Part model, mm, in its own coordinate system. A direction names the side the tool comes from. Coordinates: 2 decimals unless noted, no trailing zeros. Write each loop counter-clockwise with the first axis right and the second up, starting at its lowest first coordinate (ties: lowest second). Pieces come first, ordered by that corner, then holes. Notation, with made-up numbers: (25.25, 53.5) - (40.25, 53.5) arc R34 ccw to (40.25, 91.5) - close; hole circle Ø3 at (2, 16.5). An arc over 180 degrees is marked (long way). Write each question's results on one line, items separated by ' | '.
from build123d import *

# Parameters (mm, degrees)
F0_W      = 23
F0_H      = 18
F1_DEPTH  = 10
F2_W      = 6
F2_H      = 6
F2_H_2    = 5
F3_DEPTH  = 2.5
F4_R      = 1.19
F5_DEPTH  = 5
F6_W      = 14
F6_H      = 14
F7_DEPTH  = 5
F8_R      = 1.15
F8_R_2    = 1
F9_DEPTH  = 5
F10_W     = 23
F10_H     = 2.5
F11_DEPTH = 2


with BuildPart() as f1:
    # F0 (on Top) → F1 (new body)
    with BuildSketch(Plane.XY):
        Rectangle(F0_W, F0_H)
    extrude(amount=F1_DEPTH)

    # F2 (on face) → F3 (join)
    with BuildSketch(Plane(origin=(0, 0, 0), x_dir=(1, 0, 0), z_dir=(0, 0, -1))):
        with Locations((-8.5, 6)):
            Rectangle(F2_W, F2_H)
        with Locations((8.5, 6.5)):
            Rectangle(F2_W, F2_H_2)
    extrude(amount=F3_DEPTH)

    # F4 (on face) → F5 (join)
    with BuildSketch(Plane(origin=(0, 0, -2.5), x_dir=(1, 0, 0), z_dir=(0, 0, -1))):
        with Locations((-8.5, 6)):
            Circle(F4_R)
    extrude(amount=F5_DEPTH)

    # F6 (on face) → F7 (cut)
    with BuildSketch(Plane.XY.offset(10)):
        with Locations((0, -2)):
            Rectangle(F6_W, F6_H)
    extrude(amount=-F7_DEPTH, mode=Mode.SUBTRACT)

    # F8 (on face) → F9 (join)
    with BuildSketch(Plane.XY.offset(10)):
        with Locations((-8.9, -6.5)):
            Circle(F8_R)
        with Locations((8.9, -6.5)):
            Circle(F8_R_2)
    extrude(amount=F9_DEPTH)

    # F10 (on face) → F11 (cut)
    with BuildSketch(Plane.XY.offset(10)):
        with Locations((0, 7.75)):
            Rectangle(F10_W, F10_H)
    extrude(amount=-F11_DEPTH, mode=Mode.SUBTRACT)


solid = f1.part
(1) 3-axis set-ups, long thin cutter, end or side, ignore diameter. For faces 1 (the cylindrical face through (7.9, -6.5, 12.5)), 2 (the flat face through (0, 6.5, 9)), 3 (the flat face through (5.5, -6, -1)), 4 (the flat face through (-7, -6, -2.5)), 5 (the flat face through (0, 5, 8)): which of +Z, -Z, +X, -X, +Y, -Y reach the whole face in a straight line?
Return value:
face 1: +Z | face 2: +Z, +X, -X, +Y | face 3: -Z, +Y, -Y | face 4: -Z | face 5: +Z, -Y
(2) Saw through at B-B on x = -1. Write the cut outline in (y, z), then the cut area to 3 significant figures.
Return value:
outline: (-9, 0) - (9, 0) - (9, 8) - (6.5, 8) - (6.5, 10) - (5, 10) - (5, 5) - (-9, 5) - close | area: 105 mm^2
(3) Saw through at D-D on x = -6. Write the cut outline in (y, z).
Return value:
outline: (-9, -2.5) - (-3, -2.5) - (-3, 0) - (9, 0) - (9, 8) - (6.5, 8) - (6.5, 10) - (5, 10) - (5, 5) - (-9, 5) - close
(4) Flat gauge pins, fed straight in: P1, Ø6, axis at x = -3, y = -5.5, coming from the -Z side; P2, Ø8, axis at x = 2.5, y = 0.5, coming from the +Z side; P3, Ø8, axis at x = 5, y = -3.5, coming from the +Z side; P4, Ø0.8, axis at x = 7, z = -1, coming from the +Y side. Where does each tip first touch, or does it go through?
Return value:
P1: stops at z = -2.5 | P2: stops at z = 5 | P3: stops at z = 15 | P4: stops at y = -4
(5) Two-plate mould, pull along Y, no slides. Class faces 6 (the cylindrical face through (-9.748, -5.723, 12.465)), 7 (the flat face through (-5.5, -6, -1)), 8 (the flat face through (8, -4, -1)): released by +Y, released by -Y, zero draft, split by the parting line, or undercut.
Return value:
face 6: split by the parting line | face 7: zero draft | face 8: released by +Y
(6) Saw through at C-C on y = 5.5. Write the cut outline in (x, z), then the cut area to 3 significant figures.
Return value:
outline: (-11.5, 0) - (11.5, 0) - (11.5, 10) - (-11.5, 10) - close | area: 230 mm^2
(7) Wall check: line 1 (X direction, y = -5.75, z = -1.25); line 2 (Y direction, x = 9, z = -0.25); line 3 (Y direction, x = 1.75, z = 6.5). Give the ranges that are in metal, low to high. Write a range as from..to.
Return value:
line 1: x = -11.5..-5.5, 5.5..11.5 | line 2: y = -9..-4 | line 3: y = 5..9
(8) Saw through at A-A on z = 7. Write the cut outline in (x, y), then the cut area to 3 significant figures.
Return value:
outline: (-11.5, -9) - (-7, -9) - (-7, 5) - (7, 5) - (7, -9) - (11.5, -9) - (11.5, 9) - (-11.5, 9) - close | area: 218 mm^2
